Part model, mm, in its own coordinate system. Give positions to 0.01 mm unless a question says otherwise; leave off trailing zeros. Write each loop counter-clockwise with the first axis right and the second up, starting at its lowest first coordinate (ties: lowest second). Pieces come first, ordered by that corner, then holes.
```python
from build123d import *

# Parameters (mm, degrees)
BOSS_EXTRUDE1_DEPTH = 4.3


with BuildPart() as part:
    # Sketch1 → Boss-Extrude1 (new body)
    with BuildSketch(Plane.XY):
        with BuildLine():
            Line((-65.7, 58.81), (-65.7, -39.19))
            ThreePointArc((-65.7, -39.19), (-53.779245994, -67.969245994), (-25, -79.89))
            Line((-25, -79.89), (-0.5, -79.89))
            Line((-0.5, -79.89), (0.5, -79.89))
            Line((0.5, -79.89), (25, -79.89))
            ThreePointArc((25, -79.89), (53.779245994, -67.969245994), (65.7, -39.19))
            Line((65.7, -39.19), (65.7, 58.81))
            ThreePointArc((65.7, 58.81), (63.151828996, 64.961828996), (57, 67.51))
            Line((57, 67.51), (-57, 67.51))
            ThreePointArc((-57, 67.51), (-63.151828996, 64.961828996), (-65.7, 58.81))
        make_face()
    extrude(amount=BOSS_EXTRUDE1_DEPTH)


solid = part.part
```
1) Saw through at A-A, the plane z = 3.2. Write the cut outline in (x, y), then the cut area to 3 significant figures.
Answers follow:
outline: (-65.7, -39.19) arc R40.7 ccw to (-25, -79.89) - (25, -79.89) arc R40.7 ccw to (65.7, -39.19) - (65.7, 58.81) arc R8.7 ccw to (57, 67.51) - (-57, 67.51) arc R8.7 ccw to (-65.7, 58.81) - close
area: 18,600 mm2
2) Wall check: L1, parallel to Y at x = 30.5, z = 3.8; L2, parallel to Y at x = -45, z = 3.85; L3, parallel to X at y = 60, z = 1.1. Give the ranges that are in metal, low to high.
Answers follow:
L1: y = -79.52 to 67.51
L2: y = -74.64 to 67.51
L3: x = -65.62 to 65.62
3) Saw through at C-C, the plane x = -46.5. Write the cut outline in (y, z).
Answers follow:
outline: (-73.75, 0) - (67.51, 0) - (67.51, 4.3) - (-73.75, 4.3) - close
4) Saw through at B-B, the plane y = -62.5. Write the cut outline in (x, z).
Answers follow:
outline: (-58.36, 0) - (58.36, 0) - (58.36, 4.3) - (-58.36, 4.3) - close
5) Pin check, flat tips, straight feed: pin 1 Ø10 at (x, y) = (-19, 0.5) entering from -Z; pin 2 Ø1 at (x, z) = (51, 3.5) entering from -Y. Stop position of each tip, or through.
Answers follow:
pin 1: stops at z = 0
pin 2: stops at y = -70.91
